```python
from build123d import *

# Parameters (mm, degrees)
ESBO_O1_R                = 5.3
RESSALTO_EXTRUS_O1_DEPTH = 5
ESBO_O2_W                = 60
ESBO_O2_H                = 5
RESSALTO_EXTRUS_O2_DEPTH = 70
ESBO_O5_R                = 16
CORTE_EXTRUS_O2_DEPTH    = 2
FILETE1_R                = 5
ESBO_O3_R                = 1.75
CORTE_EXTRUS_O1_DEPTH    = 89.848185125
RESSALTO_EXTRUS_O3_DEPTH = 3
FILETE2_R                = 5
ESBO_O6_R                = 1.5
CORTE_EXTRUS_O3_DEPTH    = 89.848185125
ESBO_O8_R                = 1.5
CORTE_EXTRUS_O4_DEPTH    = 89.848185125
ESBO_O9_R                = 1.75
CORTE_EXTRUS_O5_DEPTH    = 89.848185125
ESBO_O10_R               = 1.75
CORTE_EXTRUS_O6_DEPTH    = 99.203869578
ESBO_O11_R               = 3.25
CORTE_EXTRUS_O7_DEPTH    = 2.5
ESBO_O13_W               = 13
ESBO_O13_H               = 20
ESBO_O13_R               = 1.25
RESSALTO_EXTRUS_O4_DEPTH = 18
ESBO_O18_R               = 1
CORTE_EXTRUS_O9_DEPTH    = 4
CHANFRO1_SIZE            = 2


with BuildPart() as part:
    # Esboço1 → Ressalto-extrusão1 (new body)
    with BuildSketch(Plane.XY):
        with BuildLine():
            Line((-30, 0), (-30, -37))
            Line((-30, -37), (30, -37))
            Line((30, -37), (30, 0))
            ThreePointArc((30, 0), (0, 30), (-30, 0))
        make_face()
        Circle(ESBO_O1_R, mode=Mode.SUBTRACT)
    extrude(amount=RESSALTO_EXTRUS_O1_DEPTH)

    # Esboço2 → Ressalto-extrusão2 (add)
    with BuildSketch(Plane(origin=(0, 0, 0), x_dir=(-1, 0, 0), z_dir=(0, 0, -1))):
        with Locations((0, -34.5)):
            Rectangle(ESBO_O2_W, ESBO_O2_H)
    extrude(amount=RESSALTO_EXTRUS_O2_DEPTH)

    # Esboço5 → Corte-extrusão2 (cut)
    with BuildSketch(Plane(origin=(0, 0, 0), x_dir=(-1, 0, 0), z_dir=(0, 0, -1))):
        Circle(ESBO_O5_R)
    extrude(amount=-CORTE_EXTRUS_O2_DEPTH, mode=Mode.SUBTRACT)

    # Filete1
    filete1_edges = [part.edges().sort_by_distance(p)[0] for p in [
        (30, -34.5, -70),
        (-30, -34.5, -70),
    ]]
    fillet(filete1_edges, radius=FILETE1_R)

    # Esboço3 → Corte-extrusão1 (cut, through all)
    with BuildSketch(Plane.XY.offset(5)):
        with Locations((0, 24)):
            Circle(ESBO_O3_R)
        with Locations((20.784609691, -12)):
            Circle(ESBO_O3_R)
        with Locations((-20.784609691, -12)):
            Circle(ESBO_O3_R)
    extrude(amount=-CORTE_EXTRUS_O1_DEPTH, mode=Mode.SUBTRACT)

    # Esboço4 → Ressalto-extrusão3 (add)
    with BuildSketch(Plane.ZY.offset(30)):
        Polygon((-20, -32), (0, -12), (0, -32), align=None)
    ressalto_extrus_o3 = extrude(amount=-RESSALTO_EXTRUS_O3_DEPTH)

    # Espelhar1: Ressalto-extrusão3 across plane
    add(ressalto_extrus_o3.mirror(Plane(origin=(0, 0, 0), x_dir=(0, 0, 1), z_dir=(1, 0, 0))))

    # Filete2
    filete2_edges = [part.edges().sort_by_distance(p)[0] for p in [
        (-28.5, -32, -20),
        (-28.5, -12, 0),
        (28.5, -32, -20),
        (28.5, -12, 0),
    ]]
    fillet(filete2_edges, radius=FILETE2_R)

    # Esboço6 → Corte-extrusão3 (cut, through all)
    with BuildSketch(Plane.XY.offset(5)):
        with Locations((-8, 0)):
            Circle(ESBO_O6_R)
        with Locations(Location((8, 0, 0), (0, 0, 180))):
            Circle(ESBO_O6_R)
    extrude(amount=-CORTE_EXTRUS_O3_DEPTH, mode=Mode.SUBTRACT)

    # Esboço8 → Corte-extrusão4 (cut, through all)
    with BuildSketch(Plane.XY.offset(5)):
        with Locations((0, 12)):
            Circle(ESBO_O8_R)
        with Locations(Location((0, -12, 0), (0, 0, 180))):
            Circle(ESBO_O8_R)
    extrude(amount=-CORTE_EXTRUS_O4_DEPTH, mode=Mode.SUBTRACT)

    # Esboço9 → Corte-extrusão5 (cut, through all)
    with BuildSketch(Plane.XY.offset(5)):
        with Locations((-15.5, 15.5)):
            Circle(ESBO_O9_R)
        with Locations((15.5, 15.5)):
            Circle(ESBO_O9_R)
        with Locations((15.5, -15.5)):
            Circle(ESBO_O9_R)
        with Locations((-15.5, -15.5)):
            Circle(ESBO_O9_R)
    extrude(amount=-CORTE_EXTRUS_O5_DEPTH, mode=Mode.SUBTRACT)

    # Esboço10 → Corte-extrusão6 (cut, through all)
    with BuildSketch(Plane(origin=(0, -32, 0), x_dir=(1, 0, 0), z_dir=(0, 1, 0))):
        with Locations(Location((0, 8, 0), (0, 0, 270))):
            Circle(ESBO_O10_R)
        with Locations(Location((-22, 62, 0), (0, 0, 270))):
            Circle(ESBO_O10_R)
        with Locations(Location((22, 62, 0), (0, 0, 270))):
            Circle(ESBO_O10_R)
    extrude(amount=-CORTE_EXTRUS_O6_DEPTH, mode=Mode.SUBTRACT)

    # Esboço11 → Corte-extrusão7 (cut)
    with BuildSketch(Plane(origin=(0, -32, 0), x_dir=(1, 0, 0), z_dir=(0, 1, 0))):
        with Locations(Location((-22, 62, 0), (0, 0, 270))):
            Circle(ESBO_O11_R)
        with Locations(Location((22, 62, 0), (0, 0, 270))):
            Circle(ESBO_O11_R)
        with Locations(Location((0, 8, 0), (0, 0, 270))):
            Circle(ESBO_O11_R)
    extrude(amount=-CORTE_EXTRUS_O7_DEPTH, mode=Mode.SUBTRACT)

    # Esboço13 → Ressalto-extrusão4 (add)
    with BuildSketch(Plane(origin=(0, -37, 0), x_dir=(1, 0, 0), z_dir=(0, 1, 0))):
        with Locations((-36.5, 22)):
            Rectangle(ESBO_O13_W, ESBO_O13_H)
        with Locations(Location((-36.5, 18, 0), (0, 0, 90))):
            Circle(ESBO_O13_R, mode=Mode.SUBTRACT)
        with Locations(Location((-36.5, 26, 0), (0, 0, 90))):
            Circle(ESBO_O13_R, mode=Mode.SUBTRACT)
    extrude(amount=RESSALTO_EXTRUS_O4_DEPTH)

    # Esboço18 → Corte-extrusão9 (cut)
    with BuildSketch(Plane.XY.offset(5)):
        with Locations((-7.5, -23)):
            Circle(ESBO_O18_R)
        with Locations((7.5, -23)):
            Circle(ESBO_O18_R)
    extrude(amount=-CORTE_EXTRUS_O9_DEPTH, mode=Mode.SUBTRACT)

    # Chanfro1
    # the kernel refuses this chamfer: 2 mm, written as the material it adds along each edge
    with BuildSketch(Plane(origin=(-30, -32, -16.927701836), x_dir=(0.9996219169112968, -0.027495876610585647, 0), z_dir=(0, 0, -1))) as chanfro1_piece_1:
        Polygon((CHANFRO1_SIZE * 0.999621916911, -CHANFRO1_SIZE * 0.0274958766106), (-CHANFRO1_SIZE * 0.0274958766106, -CHANFRO1_SIZE * 0.999621916911), (0, 0), align=None)
    extrude(amount=15.072298164)


solid = part.part
```
Read the model definition and answer for the solid it produces. Units are mm, in the model's axes. A direction names the side the tool comes from. Give positions to 0.01 mm unless a question says otherwise; leave off trailing zeros. Loops run counter-clockwise (first coordinate to the right, second up) from the corner with the lowest first, then second, coordinate; pieces in that order, holes last.
Item 1: For faces 5 (the cylindrical face through (-14.6, 17, 2.5)), 6 (the flat face through (-37, -28, -12)), 7 (the cylindrical face through (0.143, -33.232, -11.247)), 8 (the flat face through (-27, -26, -6)), 9 (the flat face through (4, 4, 2)), determine the directions among +Z, -Z, +X, -X, +Y, -Y from which every point of the face is accessible in a straight line to the end or side of a thin tool.
Item 2: The part is cut by section A-A (z = -8). Write down the section's boundary in (x, y), and give its area (3 significant figures).
Item 3: The mould has two halves that part along Z. Classify faces 1 (the flat face through (27, -26, -6)), 2 (the cylindrical face through (-21.857, -33.232, -65.247)), 3 (the flat face through (-23.4, -34.5, -60.6)), 4 (the flat face through (-8, -23, 1)): released by +Z, released by -Z, zero draft, split by the parting line, or undercut.
Item 4: The part is cut by section C-C (z = -30). Write down the section's boundary in (x, y), and give its area (3 significant figures).
Item 5: Find the intervals of material crossed by line 1 along X through (y, z) = (-36.5, -62); line 2 along X through (y, z) = (-15, 3); line 3 along Y through (x, z) = (0, 3), in increasing order.
Item 6: The part is cut by section D-D (y = 12). Write down the section's boundary in (x, z), and give its area (3 significant figures).
Item 7: Each of these flat-tipped pins is pushed along its axis until it touches: pin 1 Ø1.2 at (x, y) = (7.5, -23) entering from -Z; pin 2 Ø8.5 at (y, z) = (-12.5, -2) entering from -X; pin 3 Ø5.5 at (x, z) = (22, -62) entering from -Y; pin 4 Ø3 at (x, z) = (-23, -63) entering from +Y. Where does it stop, or does it pass through?
Item 8: The part is cut by section B-B (y = -4). Write down the section's boundary in (x, z).
Taken from the geometry:
1. face 5: +Z, -Z
1. face 6: +Z, -X, +Y, -Y
1. face 7: +Y
1. face 8: -Z, +Y
1. face 9: -Z
2. outline: (-30, -37) - (-1.75, -37) - (-1.75, -34.5) - (-3.25, -34.5) - (-3.25, -32) - (-27, -32) - (-27, -20) - (-30, -20) - close; (1.75, -37) - (30, -37) - (30, -20) - (27, -20) - (27, -32) - (3.25, -32) - (3.25, -34.5) - (1.75, -34.5) - close
2. area: 347 mm2
3. face 1: zero draft
3. face 2: undercut
3. face 3: undercut
3. face 4: released by +Z
4. outline: (-43, -37) - (30, -37) - (30, -32) - (-28, -32) - (-30, -30) - (-30, -19) - (-43, -19) - close
4. area: 536 mm2
5. line 1: x = -30 to -23.75, -20.25 to 20.25, 23.75 to 30
5. line 2: x = -30 to -17.18, -13.82 to 13.82, 17.18 to 30
5. line 3: y = -37 to -13.5, -10.5 to -5.3, 5.3 to 10.5, 13.5 to 22.25, 25.75 to 30
6. outline: (-27.5, 0) - (-10.58, 0) - (-10.58, 2) - (-1.5, 2) - (-1.5, 5) - (-27.5, 5) - close; (1.5, 2) - (10.58, 2) - (10.58, 0) - (27.5, 0) - (27.5, 5) - (1.5, 5) - close
6. area: 224 mm2
7. pin 1: stops at z = 0
7. pin 2: stops at x = -30
7. pin 3: stops at y = -37
7. pin 4: stops at y = -34.5
8. outline: (-30, 0) - (-15.49, 0) - (-15.49, 2) - (-3.48, 2) - (-3.48, 5) - (-30, 5) - close; (3.48, 2) - (15.49, 2) - (15.49, 0) - (30, 0) - (30, 5) - (3.48, 5) - close
